```python
from build123d import *

# Parameters (mm, degrees)
F1_DEPTH  = 50.8
F2_R      = 38.1
F3_DEPTH  = 736.6
F4_W      = 88.9
F4_H      = 298.45
F5_DEPTH  = 133.35
F7_DEPTH  = 114.3
F8_R      = 88.9
F9_DEPTH  = 177.8
F10_R     = 44.45
F11_DEPTH = 76.2
F13_DEPTH = 12.7
F14_DEPTH = 12.7
F15_R     = 28.575
F16_DEPTH = 127


with BuildPart() as f1:
    # F0 (on Top) → F1 (new body)
    with BuildSketch(Plane.XY):
        with BuildLine():
            Line((107.95, 114.3), (-107.95, 114.3))
            ThreePointArc((-107.95, 114.3), (-125.910512, 106.860512), (-133.35, 88.9))
            Line((-133.35, 88.9), (-133.35, -317.5))
            ThreePointArc((-133.35, -317.5), (-125.910512, -335.460512), (-107.95, -342.9))
            Line((-107.95, -342.9), (107.95, -342.9))
            ThreePointArc((107.95, -342.9), (125.910512, -335.460512), (133.35, -317.5))
            Line((133.35, -317.5), (133.35, 88.9))
            ThreePointArc((133.35, 88.9), (125.910512, 106.860512), (107.95, 114.3))
        make_face()
    extrude(amount=F1_DEPTH)

    # F2 (on face) → F3 (join)
    with BuildSketch(Plane.XY.offset(50.8)):
        Circle(F2_R)
    extrude(amount=F3_DEPTH)

    # F4 (on face) → F5 (join)
    with BuildSketch(Plane.XY.offset(787.4)):
        with Locations((0, -104.775)):
            Rectangle(F4_W, F4_H)
    extrude(amount=F5_DEPTH)

    # F6 (on face) → F7 (join)
    with BuildSketch(Plane.XY.offset(920.75)):
        with BuildLine():
            Line((60.96, 266.7), (-60.96, 266.7))
            ThreePointArc((-60.96, 266.7), (-87.900768, 255.540768), (-99.06, 228.6))
            Line((-99.06, 228.6), (-99.06, -285.75))
            ThreePointArc((-99.06, -285.75), (-87.900768, -312.690768), (-60.96, -323.85))
            Line((-60.96, -323.85), (60.96, -323.85))
            ThreePointArc((60.96, -323.85), (87.900768, -312.690768), (99.06, -285.75))
            Line((99.06, -285.75), (99.06, 228.6))
            ThreePointArc((99.06, 228.6), (87.900768, 255.540768), (60.96, 266.7))
        make_face()
    extrude(amount=F7_DEPTH)

    # F8 (on face) → F9 (join)
    with BuildSketch(Plane(origin=(0, 0, 920.75), x_dir=(1, 0, 0), z_dir=(0, 0, -1))):
        with Locations((0, -165.1)):
            Circle(F8_R)
    extrude(amount=F9_DEPTH)

    # F10 (on face) → F11 (join)
    with BuildSketch(Plane.YZ.offset(44.45)):
        with Locations((-184.15, 789.94)):
            Circle(F10_R)
    extrude(amount=F11_DEPTH)

    # F12 (on face) → F13 (join)
    with BuildSketch(Plane.YZ.offset(120.65)):
        Polygon((-15.997161, 700.189261), (-177.8, 793.606174), (-177.8, 980.44), (-190.5, 980.44), (-190.5, 793.606174), (-352.302839, 700.189261), (-345.952839, 689.190739), (-184.15, 782.607652), (-22.347161, 689.190739), align=None)
    extrude(amount=F13_DEPTH)

    # F12 (on face) → F14 (join)
    with BuildSketch(Plane.YZ.offset(120.65)):
        Polygon((-15.997161, 700.189261), (-177.8, 793.606174), (-177.8, 980.44), (-190.5, 980.44), (-190.5, 793.606174), (-352.302839, 700.189261), (-345.952839, 689.190739), (-184.15, 782.607652), (-22.347161, 689.190739), align=None)
    extrude(amount=F14_DEPTH)

    # F15 (on face) → F16 (join)
    with BuildSketch(Plane(origin=(0, 0, 787.4), x_dir=(1, 0, 0), z_dir=(0, 0, -1))):
        with Locations((0, 223.52)):
            Circle(F15_R)
    extrude(amount=F16_DEPTH)


solid = f1.part
```
Input: part model. Units: mm. Frame: model coordinates. A direction names the side the tool comes from. Round coordinates to 2 decimals unless told otherwise and drop trailing zeros. Loops run counter-clockwise (first coordinate to the right, second up) from the corner with the lowest first, then second, coordinate; pieces in that order, holes last. Notation, with made-up numbers: (82, -24.5) - (131, -24.5) arc R12 ccw to (131, -19.5) - close; hole circle Ø2 at (5.5, 35.25). An arc over 180 degrees is marked (long way). One line per item, written item: value. Start each with the question number.
(1) Access query for faces 4 (the flat face through (126.91, -270.27, 747.55)), 5 (the flat face through (-1, -323.85, 977)), 6 (the cylindrical face through (-19.272, 251.886, 833.095)). Directions: +Z, -Z, +X, -X, +Y, -Y. A direction counts if a zero-diameter tool reaches every point of the face in a straight line with its end or side. Return the directions, or none.
(2) Draft query along Z for faces 1 (the flat face through (-1, -24, 1035.05)), 2 (the flat face through (-44.45, -107, 853)), 3 (the cylindrical face through (125.71, -335.66, 25.04)). Return one class per face: +Z half, -Z half, draft (parallel to the pull), parting line (faces both ways), or undercut.
(3) Section D-D, the plane z = 173.5. Return loops of the section in (x, y).
(4) Contact query for flat-ended pins moving along their axis: P1, Ø4, axis at x = 124, y = -182, coming from the +Z side; P2, Ø10, axis at x = -20, z = 444, coming from the -Y side; P3, Ø10, axis at x = 86, y = -105, coming from the -Z side; P4, Ø6.5, axis at x = 126, z = 859, coming from the +Y side. Output: stop coordinate, or through.
(5) Ray query, line 1 (Z direction, x = 74.5, y = -26.5); line 2 (Z direction, x = -2.5, y = 42); line 3 (X direction, y = 31.5, z = 836.5). Return the intervals inside material, ascending. Write a range as [from, to].
(6) Section B-B, the plane x = 0. Return loops of the section in (y, z) (3 decimals), plus the area to 3 significant figures.
(7) Section A-A, the plane y = 58.5. Return loops of the section in (x, z), plus the area to 3 significant figures.
(8) Section C-C, the plane y = 165.1. Return loops of the section in (x, z).
Results below:
1. face 4: +Z, +X, -Y
1. face 5: +Z, +X, -X, -Y
1. face 6: none
2. face 1: +Z half
2. face 2: undercut
2. face 3: draft
3. outline: circle Ø76.2 at (0, 0)
4. P1: z = 980.44
4. P2: y = -35.02
4. P3: z = 0
4. P4: y = -177.8
5. line 1: [0, 50.8], [920.75, 1035.05]
5. line 2: [0, 50.8], [787.4, 1035.05]
5. line 3: [-44.45, 44.45]
6. outline: (-342.9, 0) - (114.3, 0) - (114.3, 50.8) - (38.1, 50.8) - (38.1, 787.4) - (44.45, 787.4) - (44.45, 920.75) - (76.2, 920.75) - (76.2, 742.95) - (254, 742.95) - (254, 920.75) - (266.7, 920.75) - (266.7, 1035.05) - (-323.85, 1035.05) - (-323.85, 920.75) - (-254, 920.75) - (-254, 787.4) - (-252.095, 787.4) - (-252.095, 660.4) - (-194.945, 660.4) - (-194.945, 787.4) - (-38.1, 787.4) - (-38.1, 50.8) - (-342.9, 50.8) - close
6. area: 226,000 mm^2
7. outline: (-133.35, 0) - (133.35, 0) - (133.35, 50.8) - (-133.35, 50.8) - close; (-99.06, 920.75) - (99.06, 920.75) - (99.06, 1035.05) - (-99.06, 1035.05) - close
7. area: 36,200 mm^2
8. outline: (-99.06, 920.75) - (-88.9, 920.75) - (-88.9, 742.95) - (88.9, 742.95) - (88.9, 920.75) - (99.06, 920.75) - (99.06, 1035.05) - (-99.06, 1035.05) - close
